Autodesk Inventor part; units mm, degrees
ref_plane "YZ Plane" through (0, 0, 0) normal (1, 0, 0) x (0, 1, 0)
ref_plane "XZ Plane" through (0, 0, 0) normal (0, 1, 0) x (-1, 0, 0)
ref_plane "XY Plane" through (0, 0, 0) normal (0, 0, 1) x (1, 0, 0)
sketch "Sketch1" plane through (0, 0, 0) normal (0, 0, 1) x (1, 0, 0)
  circle A0 centre (-0.7749, 5.5) radius 1
  circle A1 centre (7.2251, 5.5) radius 1
  circle A2 centre (-0.7749, -5.5) radius 1
  circle A3 centre (7.2251, -5.5) radius 1
  line L0 (11.2251, -3) -> (-3.7749, -3)
  line L1 (-3.7749, -3) -> (-3.7749, 3)
  line L2 (-3.7749, 3) -> (11.2251, 3)
  line L3 (11.2251, 3) -> (11.2251, 8)
  line L4 (11.2251, 8) -> (-8.528, 8)
  arc A4 (-8.528, -8) -> (-8.528, 8) centre (-18.7749, 0) ccw
  line L5 (-8.528, -8) -> (11.2251, -8)
  line L6 (11.2251, -8) -> (11.2251, -3)
  point P0 (0, 0)
extrude "Extrusion1" add sketch "Sketch1" along normal blind 3
sketch "Sketch2" plane through (0, 0, 3) normal (0, 0, 1) x (1, 0, 0)
  line L0 (11.2251, -8) -> (11.2251, -3)
  line L1 (11.2251, -3) -> (-3.7749, -3)
  line L2 (-3.7749, -3) -> (-3.7749, 3)
  line L3 (-3.7749, 3) -> (11.2251, 3)
  line L4 (11.2251, 3) -> (11.2251, 8)
  line L5 (11.2251, 8) -> (-8.528, 8)
  arc A0 (-8.528, -8) -> (-8.528, 8) centre (-18.7749, 0) ccw
  line L6 (-8.528, -8) -> (11.2251, -8)
  circle A1 centre (-0.7749, 5.5) radius 1
  circle A2 centre (7.2251, 5.5) radius 1
  circle A3 centre (-0.7749, -5.5) radius 1
  circle A4 centre (7.2251, -5.5) radius 1
  line L7 (11.2251, -8) -> (11.2251, -3)
  line L8 (11.2251, 3) -> (11.2251, 8)
  line L9 (11.2251, -8) -> (11.2251, 8)
  point P0 (0, 0)
extrude "Extrusion2" add sketch "Sketch2" along normal blind 5
chamfer "Chamfer1" distance 3 angle 45 1 edges at (-5.7749, 0, 8)
fillet "Fillet1" radius 1 2 edges at (-6.817, -8, 6.3872) (-6.817, 8, 6.3872)
chamfer "Chamfer2" distance 2 angle 45 1 edges at (11.2251, 0, 8)
fillet "Fillet2" radius 2 2 edges at (10.2251, -8, 7) (10.2251, 8, 7)
properties part number "armtip_2"
Read the model definition and answer for the solid it produces. Units are mm, in the model's axes. A direction names the side the tool comes from. Round coordinates to 2 decimals unless told otherwise and drop trailing zeros. Write each loop counter-clockwise with the first axis right and the second up, starting at its lowest first coordinate (ties: lowest second). Pieces come first, ordered by that corner, then holes. Notation, with made-up numbers: M -31.5,24 L -5.5,24 A11 cw -5.5,36 Z; hole C 88.25,78.5 d1. An arc over 180 degrees is marked long. Use a Markdown table: item, result.
1) Flat-ended cylindrical pins translate along their axes: pin 1 (2 mm diameter, centred on y = 1, z = 4, fed in from -X); pin 2 (0.9 mm diameter, centred on y = 0, z = 1, fed in from +X); pin 3 (3 mm diameter, centred on x = 4.5, y = -1, fed in from -Z). Find the tip coordinate at first contact, or state that the pin passes through.
Answers follow:
| item | result |
|---|---|
| pin 1 | stops at x = -5.93 |
| pin 2 | stops at x = -3.77 |
| pin 3 | stops at z = 3 |
2) The part is cut by section B-B (x = -2.25). Write down the section's boundary in (y, z).
Answers follow:
| item | result |
|---|---|
| outline | M -8,0 L -3,0 L -3,3 L 3,3 L 3,0 L 8,0 L 8,8 L -8,8 Z |
3) For a pull along X with two mould halves and no side action, classify faces 1 (the flat face through (1, 4, 0)), 2 (the cylindrical face through (-0.91, 4.51, 3.94)), 3 (the cylindrical face through (9.669, -7.626, 6.376)) as pulls with the +X half, pulls with the -X half, needs draft (parallel to the pull), parting line crosses it, or undercut.
Answers follow:
| item | result |
|---|---|
| face 1 | needs draft |
| face 2 | undercut |
| face 3 | pulls with the +X half |
4) The part is cut by section A-A (z = 1.75). Write down the section's boundary in (x, y), plus the area to 3 significant figures.
Answers follow:
| item | result |
|---|---|
| outline | M -8.53,-8 L 11.23,-8 L 11.23,-3 L -3.77,-3 L -3.77,3 L 11.23,3 L 11.23,8 L -8.53,8 A13 cw Z; hole C -0.77,-5.5 d2; hole C -0.77,5.5 d2; hole C 7.23,-5.5 d2; hole C 7.23,5.5 d2 |
| area | 183 mm2 |
5) The part is cut by section C-C (y = -5.5). Give the number of separate pieces and of enclosed holes in the cut face, plus the area to 3 significant figures.
Answers follow:
| item | result |
|---|---|
| separate pieces | 3 |
| enclosed holes | 0 |
| area | 107 mm2 |
6) A tool of negligible diameter and unlimited length cuts with its end or side. For faces 4 (the cylindrical face through (-5.775, 0.121, 2.465)), 5 (the flat face through (-3.775, 0, 1)), from which of +Z, -Z, +X, -X, +Y, -Y can it reach the whole face along a straight path? Write none if from no direction.
Answers follow:
| item | result |
|---|---|
| face 4 | +Z, -Z, -X |
| face 5 | -Z, +X |
7) Straight lines are drawn through the part: line 1 along Y through (x, z) = (6.5, 3.5); line 2 along Y through (x, z) = (7, 0.5); line 3 along X through (y, z) = (-5, 1.75). For each, find the intervals that lie inside material, in ascending order. Write a range as [from, to].
Answers follow:
| item | result |
|---|---|
| line 1 | y = [-8, -6.19], [-4.81, 4.81], [6.19, 8] |
| line 2 | y = [-8, -6.47], [-4.53, -3], [3, 4.53], [6.47, 8] |
| line 3 | x = [-6.77, -1.64], [0.09, 6.36], [8.09, 11.23] |
